from build123d import *

# Parameters (mm, degrees)
F1_DEPTH = 3.95
F2_R     = 1.9
F3_DEPTH = 3.9
F4_R     = 1


with BuildPart() as f1:
    # F0 (on Top) → F1 (new body, symmetric)
    with BuildSketch(Plane.XY):
        Polygon((0, 2.0000000475), (0, 0), (6, 0), (6, 6.5), (0, 10.1), (0, 7.740125583), (3.9123329981, 5.3927257842), (3.9123329981, 2), align=None)
        Polygon((-5.7480431453, 0), (0, 0), (0, 2.0000000475), (-3.7480431453, 2), (-3.7480431453, 5.3927257842), (0, 7.740125583), (0, 10.1), (-5.7480431453, 6.5), align=None)
    extrude(amount=F1_DEPTH, both=True)

    # F2 (on face) → F3 (join)
    with BuildSketch(Plane.XZ):
        Circle(F2_R)
    extrude(amount=F3_DEPTH)

    # F4
    f4_edges = [f1.edges().sort_by_distance(p)[0] for p in [
        (0, 10.1, 0),
        (-5.748043, 6.5, 0),
        (6, 6.5, 0),
        (-3.748043, 5.392726, 0),
        (3.912333, 5.392726, 0),
        (0, 7.740126, 0),
    ]]
    fillet(f4_edges, radius=F4_R)


solid = f1.part
Geometry check sheet. Reference: the model listing, model coordinates, mm. A direction names the side the tool comes from. Round coordinates to 2 decimals unless told otherwise and drop trailing zeros. Loops run counter-clockwise (first coordinate to the right, second up) from the corner with the lowest first, then second, coordinate; pieces in that order, holes last.
Item 1: Cross-section at B-B on y = 7.25. Record the boundary of the cut face in (x, z).
Item 2: Mould release check, pull along Y, two halves, no side actions. Record for faces 1 (the flat face through (-1.919, 6.539, 0.055)), 2 (the flat face through (0, 1.7, 3.95)), 3 (the flat face through (1, 0, 2)), 4 (the flat face through (-2.866, 8.305, 0.055)): pulls with the +Y half, pulls with the -Y half, needs draft (parallel to the pull), parting line crosses it, or undercut.
Item 3: Thickness scan on line 1 (X direction, y = 4, z = 3); line 2 (Y direction, x = 0.25, z = -2.25); line 3 (Y direction, x = 0, z = -1). Record the ranges inside material, lowest first.
Item 4: Cross-section at C-C on x = 3.75. Record the boundary of the cut face in (y, z).
Item 5: Cross-section at A-A on z = 0. Record the boundary of the cut face in (x, y), then the cut area to 3 significant figures.
Item 6: Cross-section at D-D on z = -3. Record the boundary of the cut face in (x, y), then the cut area to 3 significant figures.
Item 7: Access from +Z, -Z, +X, -X, +Y, -Y to the whole of each face (thin tool, end or side, straight path). Record for faces 5 (the cylindrical face through (-5.62, 6.44, -0.06)), 6 (the cylindrical face through (-1.9, -1.92, 0.08)), 7 (the flat face through (1.956, 6.567, 0.055)).
Item 8: Gauge pin test, flat ends, axial feed: pin 1 (4 mm diameter, centred on x = -2, z = -1, fed in from -Y); pin 2 (1.9 mm diameter, centred on x = -1.5, z = -1.5, fed in from +Y). Record the tip position at first contact, or that the pin passes through.
Answer sheet:
1. outline: (-4.55, -3.95) - (-0.78, -3.95) - (-0.78, 3.95) - (-4.55, 3.95) - close; (0.82, -3.95) - (4.75, -3.95) - (4.75, 3.95) - (0.82, 3.95) - close
2. face 1: undercut
2. face 2: needs draft
2. face 3: pulls with the -Y half
2. face 4: pulls with the +Y half
3. line 1: x = -5.75 to -3.75, 3.91 to 6
3. line 2: y = 0 to 2, 7.54 to 9.9
3. line 3: y = -3.9 to 2, 7.57 to 9.93
4. outline: (0, -3.95) - (2, -3.95) - (2, 3.95) - (0, 3.95) - close; (5.37, -3.95) - (7.85, -3.95) - (7.85, 3.95) - (5.37, 3.95) - close
5. outline: (-5.75, 0) - (-1.9, 0) - (-1.9, -3.9) - (1.9, -3.9) - (1.9, 0) - (6, 0) - (6, 5.93) arc R1 ccw to (5.51, 6.79) - (0.53, 9.78) arc R1 ccw to (-0.52, 9.77) - (-5.28, 6.79) arc R1 ccw to (-5.75, 5.95) - close; hole (-3.75, 2) - (3.91, 2) - (3.91, 4.83) arc R1 ccw to (3.43, 5.68) - (0.53, 7.42) arc R1 ccw to (-0.52, 7.41) - (-3.28, 5.69) arc R1 ccw to (-3.75, 4.84) - close
5. area: 77.3 mm2
6. outline: (-5.75, 0) - (6, 0) - (6, 5.93) arc R1 ccw to (5.51, 6.79) - (0.53, 9.78) arc R1 ccw to (-0.52, 9.77) - (-5.28, 6.79) arc R1 ccw to (-5.75, 5.95) - close; hole (-3.75, 2) - (3.91, 2) - (3.91, 4.83) arc R1 ccw to (3.43, 5.68) - (0.53, 7.42) arc R1 ccw to (-0.52, 7.41) - (-3.28, 5.69) arc R1 ccw to (-3.75, 4.84) - close
6. area: 62.5 mm2
7. face 5: +Z, -Z, -X, +Y
7. face 6: -Y
7. face 7: +Z, -Z
8. pin 1: stops at y = -3.9
8. pin 2: stops at y = 9.76
